Could you check a few things on this model? Use its own coordinates, in mm. A direction names the side the tool comes from. Coordinates: 2 decimals unless noted, no trailing zeros. Loops run counter-clockwise (first coordinate to the right, second up) from the corner with the lowest first, then second, coordinate; pieces in that order, holes last. Notation, with made-up numbers: (-39.5, -5.75) - (-4.5, -5.75) arc R22 ccw to (-4.5, 28.25) - close; hole circle Ø6 at (-13.5, -14). An arc over 180 degrees is marked (long way). Use CSV: the item, a comma, the result in double quotes.
Autodesk Inventor part; units mm, degrees
ref_plane "YZ Plane" through (0, 0, 0) normal (1, 0, 0) x (0, 1, 0)
ref_plane "XZ Plane" through (0, 0, 0) normal (0, 1, 0) x (-1, 0, 0)
ref_plane "XY Plane" through (0, 0, 0) normal (0, 0, 1) x (1, 0, 0)
ref_plane "Arbeitsebene1" through (0, 0, -8) normal (0, 0, -1) x (-1, 0, 0)
sketch "Skizze1" plane through (0, 0, -8) normal (0, 0, -1) x (-1, 0, 0)
  line L0 (-30, -73.2876) -> (-18.6416, -61.9292)
  line L1 (-18.6416, -61.9292) -> (-17.5809, -62.9898)
  line L2 (-17.5809, -62.9898) -> (-30, -75.4089)
  line L3 (-30, -75.4089) -> (-30, -76)
  arc A0 (-30, -76) -> (-26, -80) centre (-26, -76) ccw
  line L4 (-18, -80) -> (-26, -80)
  arc A1 (-18, -80) -> (-14, -76) centre (-18, -76) ccw
  line L5 (-14, -34) -> (-14, -76)
  arc A2 (-10, -30) -> (-14, -34) centre (-10, -34) ccw
  line L6 (-10, -30) -> (12, -30)
  arc A3 (16, -34) -> (12, -30) centre (12, -34) ccw
  line L7 (16, -34) -> (16, -76)
  arc A4 (16, -76) -> (20, -80) centre (20, -76) ccw
  line L8 (20, -80) -> (26, -80)
  arc A5 (26, -80) -> (30, -76) centre (26, -76) ccw
  line L9 (30, 28) -> (30, -76)
  line L10 (30, 28) -> (28, 30)
  line L11 (28, 30) -> (-28, 30)
  line L12 (-28, 30) -> (-30, 28)
  line L13 (-30, 28) -> (-30, -73.2876)
  circle A6 centre (-10, -25) radius 1.45
  circle A7 centre (-10, 25) radius 1.45
  circle A8 centre (10, 25) radius 1.45
  circle A9 centre (10, -25) radius 1.45
  circle A10 centre (25, -10) radius 1.45
  circle A11 centre (-25, -10) radius 1.45
  circle A12 centre (-25, 10) radius 1.45
  circle A13 centre (25, 10) radius 1.45
  circle A14 centre (-17.5, -17.5) radius 1.95
  circle A15 centre (17.5, 17.5) radius 1.95
  circle A16 centre (17.5, -17.5) radius 1.95
  circle A17 centre (-17.5, 17.5) radius 1.95
  circle A18 centre (-25, 25) radius 2.325
  circle A19 centre (25, -25) radius 2.325
  circle A20 centre (-25, -25) radius 2.325
  circle A21 centre (25, 25) radius 2.325
  circle A22 centre (0, 0) radius 16
  circle A23 centre (23, -74) radius 3.75
  circle A24 centre (23, -64) radius 1.45
  circle A25 centre (23, -54) radius 1.45
  line L14 (7, -80) -> (39, -80)
  line L15 (39, -80) -> (39, -48)
  line L16 (39, -48) -> (7, -48)
  line L17 (7, -48) -> (7, -80)
  line L18 (7, -80) -> (39, -48) construction
  line L19 (39, -80) -> (7, -48) construction
  circle A26 centre (23, -74) radius 1.4
  line L20 (34.516, -58.7768) -> (32.4244, -50.9708)
  line L21 (24.0592, -48.7293) -> (7.7293, -65.0592)
  line L22 (9.9708, -73.4244) -> (17.7768, -75.516)
  circle A27 centre (24.1439, -65.1439) radius 11.6667
  arc A28 (7.7293, -65.0592) -> (9.9708, -73.4244) centre (11.2649, -68.5948) ccw
  line L23 (34.516, -58.7768) -> (17.7768, -75.516)
  arc A29 (32.4244, -50.9708) -> (24.0592, -48.7293) centre (27.5948, -52.2649) ccw
  point P0 (0, 0)
  point P1 (26, -80)
  point P2 (16, -48)
  point P3 (16, -56.7886)
  point P4 (19.8793, -76.0794)
  point P5 (24.6629, -77.3611)
  point P6 (24.985, -48)
  point P7 (7, -65.985)
  point P8 (7, -71.2045)
  point P9 (30.2045, -48)
  dimension "d0" = 32
  dimension "d1" = 32
  dimension "d2" = 2.8
extrude "Extrusion1" add sketch "Skizze1" along normal blind 32 contours L16 A29 L20 L23 A27 L9 | L9 A27 A25 L21 A29 L16 | L16 L15 L14 A5 L9 A27 L23 L20 A29 | A29 L21 L7 L16 | A27 L23 L9 | L9 L23 A23 A27 L7 A25 | L7 L21 A28 L17 L16 | L23 A27 L9 | L9 A27 A23 L23 | A27 L7 L22 A28 L17 L21 | L7 A27 | L9 A5 L8 A4 L7 L22 L23 A27 A23 | L23 A23 | A23 A27 L23 | A27 L23 L22 L7 | A23 A27 | A23 A27 L23 | L14 L17 A28 L22 L7 A4
sketch "Skizze2" plane through (0, 0, -8) normal (0, 0, -1) x (-1, 0, 0)
  circle A0 centre (33.5719, -74.5719) radius 1.4
  line L0 (33.5719, -74.5719) -> (11.2649, -68.5948)
  line L1 (11.2649, -68.5948) -> (27.5948, -52.2649)
  line L2 (27.5948, -52.2649) -> (33.5719, -74.5719)
  line L3 (9.7029, -90.6426) -> (49.4807, -50.8648) construction
  line L4 (-4.7029, -89.492) -> (48.3301, -36.459) construction
  line L5 (39, -80) -> (39, -48) construction
  line L6 (7, -48) -> (7, -80) construction
  line L7 (39, -80) -> (7, -48) construction
  arc A1 (32.4244, -50.9708) -> (24.0592, -48.7293) centre (27.5948, -52.2649) ccw
  line L8 (24.0592, -48.7293) -> (7.7293, -65.0592)
  arc A2 (7.7293, -65.0592) -> (9.9708, -73.4244) centre (11.2649, -68.5948) ccw
  line L9 (9.9708, -73.4244) -> (32.2778, -79.4016)
  arc A3 (32.2778, -79.4016) -> (38.4016, -73.2778) centre (33.5719, -74.5719) ccw
  line L10 (38.4016, -73.2778) -> (32.4244, -50.9708)
  point P0 (0, 0)
  point P1 (24.4298, -55.4298)
  point P2 (24.1439, -65.1439)
hole "Bohrung1" at (-27.5948, -52.2649, -8) at (-11.2649, -68.5948, -8) at (-33.5719, -74.5719, -8) direction (0, 0, -1) diameter 2.8 end through all counterbore diameter 6 counterbore depth 25
sketch "Skizze4" plane through (-32.4244, -50.9708, -40) normal (-0.9659, 0.2588, 0) x (0, 0, 1)
  line L0 (6.9, -13.047) -> (-22.6933, -13.047)
  line L1 (6.9, -10.047) -> (-22.6933, -10.047)
  circle A0 centre (4.5207, -11.5212) radius 1.4
  point P0 (40, 57.626)
  dimension "d19" = 2.8
extrude "Extrusion3" [suppressed]
sketch "Skizze5" plane through (0, 0, -40) normal (0, 0, -1) x (-1, 0, 0)
  line L0 (9.9708, -73.4244) -> (17.7768, -75.516)
  line L1 (24.0592, -48.7293) -> (7.7293, -65.0592)
  line L2 (34.516, -58.7768) -> (32.4244, -50.9708)
  circle A0 centre (24.1439, -65.1439) radius 11.6667
  circle A1 centre (24.1439, -65.1439) radius 0.5
  point P0 (0, 0)
  dimension "d22" = 1
extrude "Extrusion4" cut sketch "Skizze5" against normal blind 1 contours A1
pattern_circular "Runde Anordnung2" [suppressed]
properties part number "30_XY_Sample_lightsheetarm_sample_screwadapter_v3"
(1) Suppose I cut it at B-B (y = -64). Write out the boundary of the cut face in (x, z), plus the area to 3 significant figures.
Computed:
outline,"(-39, -40) - (-24.45, -40) - (-24.45, -8) - (-39, -8) - close; (-21.55, -40) - (-7, -40) - (-7, -8) - (-21.55, -8) - close"
area,"931 mm²"
(2) Will these pins go through, and if not, where does the flat tip stop? pin 1 (4.5 mm diameter, centred on x = -33.57, y = -74.57, fed in from -Z); pin 2 (5 mm diameter, centred on x = -28, y = -52.5, fed in from +Z).
Computed:
pin 1,"stops at z = -40"
pin 2,"stops at z = -33"
(3) Which directions (+Z, -Z, +X, -X, +Y, -Y) give clear straight access to the entire face, cutting with the end or side of a thin tool? Please do faces 4 (the face through (-24.487, -65.508, -39.507)), 5 (the face through (-34.52, -73.54, -36.55)), 6 (the face through (-31.75, -72.19, -20.68)).
Computed:
face 4,"-Z"
face 5,"+Z, -Z"
face 6,"+Z"
(4) Thinking about a two-plate mould opening in Y: for faces 1 (the face through (-13.29, -66.38, -20.68)), 2 (the face through (-7, -64, -24)), 3 (the face through (-23, -80, -24)), which applies, +Y half, -Y half, draft (parallel to the pull), parting line (faces both ways), or undercut?
Computed:
face 1,"undercut"
face 2,"draft"
face 3,"-Y half"
(5) Please list where these lines run through material, in increasing order: line 1 (Y direction, x = -23, z = -25); line 2 (X direction, y = -54, z = -20); line 3 (X direction, y = -74, z = -15).
Computed:
line 1,"y = -80 to -75.4, -72.6 to -65.45, -62.55 to -55.45, -52.55 to -48"
line 2,"x = -39 to -30.04, -25.15 to -24.45, -21.55 to -7"
line 3,"x = -39 to -36.52, -30.63 to -24.4, -21.6 to -7"
(6) Suppose I cut it at A-A (x = -23). Write out the boundary of the cut face in (y, z), plus the area to 3 significant figures.
Computed:
outline,"(-80, -40) - (-75.4, -40) - (-75.4, -8) - (-80, -8) - close; (-72.6, -40) - (-65.45, -40) - (-65.45, -8) - (-72.6, -8) - close; (-62.55, -40) - (-55.45, -40) - (-55.45, -8) - (-62.55, -8) - close; (-52.55, -40) - (-48, -40) - (-48, -8) - (-52.55, -8) - close"
area,"749 mm²"
(7) Suppose I cut it at C-C (x = -10.5). Write out the boundary of the cut face in (y, z), plus the area to 3 significant figures.
Computed:
outline,"(-80, -40) - (-69.77, -40) - (-69.77, -33) - (-71.5, -33) - (-71.5, -8) - (-80, -8) - close; (-67.42, -40) - (-48, -40) - (-48, -8) - (-65.69, -8) - (-65.69, -33) - (-67.42, -33) - close"
area,"863 mm²"
(8) Suppose I cut it at D-D (z = -34). Write out the boundary of the cut face in (x, y), plus the area to 3 significant figures.
Computed:
outline,"(-39, -80) - (-7, -80) - (-7, -48) - (-39, -48) - close; hole circle Ø2.8 at (-33.57, -74.57); hole circle Ø2.8 at (-27.59, -52.26); hole circle Ø2.9 at (-23, -64); hole circle Ø2.9 at (-23, -54); hole circle Ø2.8 at (-23, -74); hole circle Ø2.8 at (-11.26, -68.59)"
area,"986 mm²"
